Autodesk Inventor part; units mm, degrees
ref_plane "WeldJoint" through (0, 0, -10) normal (0.5299, -0.848, 0) x (0, 0, 1)
ref_plane "Outer" through (0, 0, -10) normal (0.454, -0.891, 0) x (0, 0, 1)
ref_plane "Clock_Feeder" through (0, 0, -10) normal (0.7071, 0.7071, 0) x (0, 0, 1)
sketch "Sketch13" plane through (0, 0, 0) normal (0, 0, 1) x (1, 0, 0)
  circle A0 centre (0, 0) radius 476 construction
  line L0 (0, 0) -> (0, -476)
  line L1 (0, 0) -> (-403.6709, -252.2416)
  line L2 (0, 0) -> (336.5828, -336.5828)
  line L3 (0, 0) -> (0, -476)
  line L4 (0, 0) -> (0, -476)
  line L5 (0, 0) -> (-424.1191, -216.0995)
  arc A1 (-403.6709, -252.2416) -> (0, -476) centre (0, 0) ccw
  dimension "d53" = 952
  dimension "d54" = 58
  dimension "d55" = 0
  dimension "d56" = 0
  dimension "d57" = 315
  dimension "d58" = 63
ref_plane "WeldJoint" through (0, 0, -10) normal (0.5299, -0.848, 0) x (0, 0, 1)
ref_plane "Outer" through (0, 0, -10) normal (0.454, -0.891, 0) x (0, 0, 1)
ref_plane "Clock_Feeder" through (0, 0, -10) normal (0.7071, 0.7071, 0) x (0, 0, 1)
ref_plane "Charging" through (0, 0, -10) normal (1, 0, 0) x (0, 0, 1)
ref_plane "Accsess" through (0, 0, -10) normal (1, 0, 0) x (0, 0, 1)
sketch "Sketch14" plane through (0, 0, -10) normal (0.5299, -0.848, 0) x (0, 0, 1)
  line L0 (1510, 470) -> (10, 470)
  line L1 (10, 470) -> (10, 476)
  line L2 (10, 476) -> (1510, 476)
  line L3 (1510, 476) -> (1510, 470)
  line L4 (10, 0) -> (825.0673, 0)
  point P0 (10, 473)
  dimension "d59" = 1500
  dimension "d60" = 6
  dimension "d61" = 952
revolve "Revolution2" add sketch "Sketch14" angle 359.9 about axis through (0, 0, 0) along (0, 0, 1)
sketch "Sketch AnglePlane_Feeder" plane through (0, 0, -10) normal (0.7071, 0.7071, 0) x (0, 0, 1)
  line L0 (10, -476) -> (10, 476)
  line L1 (10, 0) -> (1210, 0)
  line L2 (1210, 0) -> (1210, 476)
  line L3 (1210, 476) -> (10, 476)
  line L4 (10, 476) -> (10, 0)
  point P0 (10, -107.0767)
  point P1 (10, -107.886)
  dimension "d63" = 952
  dimension "d64" = 90
  dimension "frd_hght" = 1200
ref_plane "AnglePlane_Feeder" through (0, 0, 1200) normal (0.7071, -0.7071, 0) x (0.7071, 0.7071, 0)
sketch "Sketch16" plane through (0, 0, 1200) normal (0.7071, -0.7071, 0) x (0.7071, 0.7071, 0)
  circle A0 centre (0, 0) radius 45.5
  point P0 (0, -1200)
  point P1 (0, 0)
  point P2 (0, 0)
  point P3 (0, 0)
  dimension "d66" = 91
extrude "Extrusion7" cut sketch "Sketch16" along normal through all
ref_plane "Work Plane16" through (0, 0, 0) normal (0, -1, 0) x (1, 0, 0)
sketch "Sketch17" plane through (0, 0, 0) normal (0, -1, 0) x (1, 0, 0)
  circle A0 centre (0, 408.5) radius 268.5
  line L0 (0, 140) -> (-495.5727, 140)
  point P0 (0, 0)
  dimension "d69" = 537
  dimension "d71" = 140
extrude "Extrusion8" cut sketch "Sketch17" along normal through all
sketch "Sketch19" plane through (0, 0, -10) normal (1, 0, 0) x (0, 0, 1)
  line L0 (10, 0) -> (1260, 0)
  line L1 (1260, 0) -> (1260, 476)
  line L2 (1260, 476) -> (10, 476)
  line L3 (10, 476) -> (10, 0)
  dimension "d74" = 1250
  dimension "d76" = 952
  dimension "d77" = 90
ref_plane "Work Plane18" through (0, 0, 1250) normal (0, -1, 0) x (1, 0, 0)
sketch "Sketch20" plane through (0, 0, 1250) normal (0, -1, 0) x (1, 0, 0)
  line L0 (-103.5, 0) -> (103.5, 0)
  line L1 (103.5, 0) -> (103.5, 125)
  line L2 (103.5, 125) -> (-103.5, 125)
  line L3 (-103.5, 125) -> (-103.5, 0)
  point P0 (0, -1250)
  point P1 (0, 0)
  point P2 (0, 0)
  point P3 (0, 0)
  point P4 (0, 0)
  dimension "d78" = 207
  dimension "d79" = 125
extrude "Extrusion9" cut sketch "Sketch20" along normal through all
equation "\"BendRadius\" = Thickness"
equation "\"BendReliefWidth\" = Thickness"
equation "\"BendReliefDepth\" = 0.5 * Thickness"
equation "\"CornerReliefSize\" = 4 * Thickness"
equation "\"MinimumRemnant\" = 2 * Thickness"
equation "\"TransitionRadius\" = BendRadius"
equation "\"JacobiRadiusSize\" = BendRadius"
equation "\"GapSize\" = Thickness"
equation "\"Feeder_horisont_angle\" = 0"
equation "\"MAIN_filter_diam\" = 952"
equation "\"Hatch_Accsess_diameter\" = 535"
equation "\"Clock_Accsess_angle\" = 0"
equation "\"Clock_Charging_agnle\" = 0"
equation "\"Clock_Feeder_angle\" = 315deg"
equation "\"Clock_Outer_angle\" = 63deg"
equation "\"Clock_WeldJoint_angle\" = 58deg"
properties part number "PNS 9110 main Shell D 940" material "Steel"
Part model, mm, in its own coordinate system. Round coordinates to 2 decimals unless told otherwise and drop trailing zeros. Loops run counter-clockwise (first coordinate to the right, second up) from the corner with the lowest first, then second, coordinate; pieces in that order, holes last. Notation, with made-up numbers: (-15, -7.75) -> (-3, -7.75) arc R11 cw to (-3, 1.25) -> close; hole circle Ø6 at (-15.5, 0). An arc over 180 degrees is marked (long way). Use one line per item in the form item = value. Start each with the question number.
Item 1: Two-plate mould, pull along X, no slides. Class faces 1 (the cylindrical face through (-208.191, -427.33, 578.055)), 2 (the cylindrical face through (308.11, -359.17, 1227.69)), 3 (the cylindrical face through (167.324, 445.622, 760.5)), 4 (the flat face through (-453, 130, 0)): released by +X, released by -X, zero draft, split by the parting line, or undercut.
Item 2: Drop flat-ended pins along their axis: pin 1 Ø5.5 at (x, y) = (-26, -465) entering from -Z; pin 2 Ø8 at (x, z) = (-365.5, 769) entering from +Y; pin 3 Ø4 at (y, z) = (109.5, 419) entering from +X; pin 4 Ø12 at (y, z) = (260, 1145) entering from -X. Give the stop position or say it passes through.
Item 3: Band-saw the part on B-B (x = 0). List the corners of the cut face in (y, z).
Item 4: Band-saw the part on A-A (y = 0). List the corners of the cut face in (x, z), plus the area to 3 significant figures.
Item 5: Band-saw the part on C-C (z = 1276). List the corners of the cut face in (x, y).
Item 6: Drill centre lines: line 1 along X through (y, z) = (0, 1098); line 2 along X through (y, z) = (-17.5, 919.5). Where is each one in solid material? Low to high.
Item 7: Band-saw the part on D-D (z = 829). List the corners of the cut face in (x, y).
Data:
q1.face_1 = undercut
q1.face_2 = undercut
q1.face_3 = split by the parting line
q1.face_4 = zero draft
q2.pin_1 = through
q2.pin_2 = 309.67
q2.pin_3 = 463.7
q2.pin_4 = -402.57
q3.outline = (-476, 0) -> (-470, 0) -> (-470, 140) -> (-476, 140) -> close; (-476, 677) -> (-470, 677) -> (-470, 1250) -> (-476, 1250) -> close; (-476, 1375) -> (-470, 1375) -> (-470, 1500) -> (-476, 1500) -> close; (470, 0) -> (476, 0) -> (476, 1500) -> (470, 1500) -> close
q4.outline = (-476, 0) -> (-470, 0) -> (-470, 1500) -> (-476, 1500) -> close; (470, 0) -> (476, 0) -> (476, 1500) -> (470, 1500) -> close
q4.area = 18,000 mm^2
q5.outline = (-404.11, -251.54) -> (-399.02, -248.37) arc R470 cw (long way) to (103.5, -458.46) -> (103.5, -464.61) arc R476 ccw (long way) to start; (-403.67, -252.24) arc R476 ccw to (-103.5, -464.61) -> (-103.5, -458.46) arc R470 cw to (-398.58, -249.06) -> close
q6.line_1 = -476 to -470, 470 to 476
q6.line_2 = -475.68 to -469.67, 469.67 to 475.68
q7.outline = (-404.11, -251.54) -> (-399.02, -248.37) arc R470 cw (long way) to (-398.58, -249.06) -> (-403.67, -252.24) arc R476 ccw (long way) to start
